Build history of the part. All positions in model axes, mm. A direction names the side the tool comes from. Coordinates: 2 decimals unless noted, no trailing zeros. Loops run counter-clockwise (first coordinate to the right, second up) from the corner with the lowest first, then second, coordinate; pieces in that order, holes last.
Item 1: Mould opens along Z. For faces 1 (the face through (-20, -10, 10)), 2 (the face through (-19, 0, 8)), 3 (the face through (-15, -10, 0)) say: released by +Z, released by -Z, zero draft, split by the parting line, or undercut.
Item 2: 3-axis set-ups, long thin cutter, end or side, ignore diameter. For faces 4 (the face through (-30, -10, 8)), 5 (the face through (-25, -5, 13)), 6 (the face through (-5, -10, 3)): which of +Z, -Z, +X, -X, +Y, -Y reach the whole face in a straight line?
Item 3: Cut at D-D (y = -7). List the corners of the cut face in (x, z), and give its area (3 significant figures).
Item 4: Flat gauge pins, fed straight in: pin 1 (2 mm diameter, centred on y = -11.5, z = 2.5, fed in from +X); pin 2 (3 mm diameter, centred on y = -7.5, z = 17, fed in from -X); pin 3 (5 mm diameter, centred on x = -24.5, y = -8, fed in from +Z). Where does each tip first touch, or does it go through?
Item 5: Drill centre lines: line 1 along Z through (x, y) = (-28, -10.5); line 2 along Y through (x, z) = (-25, 11.75); line 3 along X through (y, z) = (-7.25, 7). Where is each one in solid material? Low to high.
Item 6: Cut at C-C (z = 1.5). List the corners of the cut face in (x, y), and give its area (3 significant figures).
Item 7: Cut at A-A (z = 12.25). List the corners of the cut face in (x, y).
Item 8: Cut at B-B (x = -15.5). List the corners of the cut face in (y, z), and give its area (3 significant figures).
from build123d import *

# Parameters (mm, degrees)
F1_DEPTH = 20
F2_W     = 10
F2_H     = 10
F3_DEPTH = 30.001
F4_W     = 5
F4_H     = 10
F5_DEPTH = 25


with BuildPart() as f1:
    # F0 (on Front) → F1 (new body)
    with BuildSketch(Plane.XZ):
        Polygon((0, 4.166667), (-30, 20), (-30, 0), (0, 0), align=None)
    extrude(amount=F1_DEPTH)

    # F2 (on Right) → F3 (cut, through all)
    with BuildSketch(Plane.YZ):
        with Locations((-10, 15)):
            Rectangle(F2_W, F2_H)
    extrude(amount=-F3_DEPTH, mode=Mode.SUBTRACT)

    # F4 (on face) → F5 (cut)
    with BuildSketch(Plane(origin=(0, 0, 0), x_dir=(1, 0, 0), z_dir=(0, 0, -1))):
        with Locations((-2.5, 10)):
            Rectangle(F4_W, F4_H)
    extrude(amount=-F5_DEPTH, mode=Mode.SUBTRACT)


solid = f1.part
Filled sheet:
1. face 1: released by +Z
1. face 2: zero draft
1. face 3: released by -Z
2. face 4: +Z, -Z, -X, +Y, -Y
2. face 5: +Z, +X, -X
2. face 6: +Z, -Z, +X
3. outline: (-30, 0) - (-5, 0) - (-5, 6.81) - (-11.05, 10) - (-30, 10) - close
3. area: 240 mm2
4. pin 1: stops at x = -5
4. pin 2: passes through
4. pin 3: stops at z = 10
5. line 1: z = 0 to 10
5. line 2: y = -20 to -15, -5 to 0
5. line 3: x = -30 to -5.37
6. outline: (-30, -20) - (0, -20) - (0, -15) - (-5, -15) - (-5, -5) - (0, -5) - (0, 0) - (-30, 0) - close
6. area: 550 mm2
7. outline: (-30, -20) - (-15.32, -20) - (-15.32, -15) - (-30, -15) - close; (-30, -5) - (-15.32, -5) - (-15.32, 0) - (-30, 0) - close
8. outline: (-20, 0) - (0, 0) - (0, 12.35) - (-5, 12.35) - (-5, 10) - (-15, 10) - (-15, 12.35) - (-20, 12.35) - close
8. area: 223 mm2
